```python
from build123d import *

# Parameters (mm, degrees)
SKETCH1_W           = 58.42
SKETCH1_H           = 58.42
BOSS_EXTRUDE1_DEPTH = 56
SKETCH2_R           = 30
BOSS_EXTRUDE2_DEPTH = 72
SKETCH3_R           = 6
BOSS_EXTRUDE3_DEPTH = 30
SKETCH4_R           = 2.5
CUT_EXTRUDE1_DEPTH  = 25.4
SKETCH5_W           = 2.5
SKETCH5_H           = 4
CUT_EXTRUDE2_DEPTH  = 18.8
SKETCH6_R           = 16
BOSS_EXTRUDE4_DEPTH = 2
CUT_EXTRUDE3_REACH  = 28.5


with BuildPart() as part:
    # Sketch1 → Boss-Extrude1 (new body)
    with BuildSketch(Plane(origin=(0, 0, 0), x_dir=(1, 0, 0), z_dir=(0, 1, 0))):
        Rectangle(SKETCH1_W, SKETCH1_H)
    extrude(amount=BOSS_EXTRUDE1_DEPTH)

    # Sketch2 → Boss-Extrude2 (add)
    with BuildSketch(Plane(origin=(0, 56, 0), x_dir=(1, 0, 0), z_dir=(0, 1, 0))):
        Circle(SKETCH2_R)
    extrude(amount=BOSS_EXTRUDE2_DEPTH)

    # Sketch3 → Boss-Extrude3 (add)
    with BuildSketch(Plane(origin=(0, 128, 0), x_dir=(1, 0, 0), z_dir=(0, 1, 0))):
        Circle(SKETCH3_R)
    extrude(amount=BOSS_EXTRUDE3_DEPTH)

    # Sketch4 → Cut-Extrude1 (cut)
    with BuildSketch(Plane(origin=(0, 128, 0), x_dir=(1, 0, 0), z_dir=(0, 1, 0))):
        with Locations((-15.909902577, 15.909902577)):
            Circle(SKETCH4_R)
        with Locations((15.909902577, 15.909902577)):
            Circle(SKETCH4_R)
        with Locations((15.909902577, -15.909902577)):
            Circle(SKETCH4_R)
        with Locations((-15.909902577, -15.909902577)):
            Circle(SKETCH4_R)
    extrude(amount=-CUT_EXTRUDE1_DEPTH, mode=Mode.SUBTRACT)

    # Sketch5 → Cut-Extrude2 (cut)
    with BuildSketch(Plane(origin=(0, 158, 0), x_dir=(1, 0, 0), z_dir=(0, 1, 0))):
        with Locations((4.75, 0)):
            Rectangle(SKETCH5_W, SKETCH5_H)
    extrude(amount=-CUT_EXTRUDE2_DEPTH, mode=Mode.SUBTRACT)

    # Sketch6 → Boss-Extrude4 (add)
    with BuildSketch(Plane(origin=(0, 128, 0), x_dir=(1, 0, 0), z_dir=(0, 1, 0))):
        Circle(SKETCH6_R)
    extrude(amount=BOSS_EXTRUDE4_DEPTH)

    # Sketch7 → Cut-Extrude3 (cut, up to next)
    with BuildSketch(Plane(origin=(3.5, 0, 0), x_dir=(0, 0, -1), z_dir=(1, 0, 0)), mode=Mode.PRIVATE) as cut_extrude3_sk1:
        with BuildLine():
            Line((2, 139.2), (-2, 139.2))
            ThreePointArc((-2, 139.2), (0, 137.2), (2, 139.2))
        make_face()
    cut_extrude3_tool1 = extrude(cut_extrude3_sk1.sketch, amount=CUT_EXTRUDE3_REACH, mode=Mode.PRIVATE) & part.part
    add(cut_extrude3_tool1.solids().sort_by_distance((3.5, 138.351174, 0))[0], mode=Mode.SUBTRACT)


solid = part.part
```
Input: part model. Units: mm. Frame: model coordinates. A direction names the side the tool comes from. Coordinates: 2 decimals unless noted, no trailing zeros. Loops run counter-clockwise (first coordinate to the right, second up) from the corner with the lowest first, then second, coordinate; pieces in that order, holes last. Notation, with made-up numbers: M 62,19 L 112,19 A24 ccw 112,34 Z; hole C 10,65 d4. An arc over 180 degrees is marked long. One line per item, written item: value.
(1) Pin query (flat end, axial travel): pin 1 (4 mm diameter, centred on x = -15.5, y = 93, fed in from +Z); pin 2 (10 mm diameter, centred on x = 7.5, y = 87.5, fed in from -Z); pin 3 (1.2 mm diameter, centred on y = 147.5, z = 1, fed in from +X). Return the tip coordinate at first contact, or that it passes through.
Filled in:
pin 1: z = 26.79
pin 2: z = -29.9
pin 3: x = 3.5
(2) Section A-A (z = 0). Output: boundary loops of the cut face in (x, y), and give its area (3 significant figures).
Filled in:
outline: M -30,56 L -29.21,56 L -29.21,0 L 29.21,0 L 29.21,56 L 30,56 L 30,128 L 16,128 L 16,130 L 6,130 L 6,137.2 L 3.5,137.2 L 3.5,158 L -6,158 L -6,130 L -16,130 L -16,128 L -30,128 Z
area: 7,940 mm^2
(3) Section C-C (y = 23). Output: boundary loops of the cut face in (x, z).
Filled in:
outline: M -29.21,-29.21 L 29.21,-29.21 L 29.21,29.21 L -29.21,29.21 Z
(4) Line query: line 1 along Z through (x, y) = (10, 37.5); line 2 along Z through (x, y) = (14.5, 111); line 3 along Y through (x, z) = (23, -24). Output: solid intervals per line, ascending. Write a range as from..to.
Filled in:
line 1: -29.21..29.21
line 2: -26.26..-17.97, -13.85..13.85, 17.97..26.26
line 3: 0..56
(5) Pull-direction query (X, two-part tool) for faces 1 (the flat face through (3.5, 148, 0)), 2 (the flat face through (13, 128, 13)), 3 (the cylindrical face through (-4.76, 143.8, 3.65)), 4 (the flat face through (-16, 102.6, -16)); classes: +X half, -X half, draft (parallel to the pull), parting line (faces both ways), or undercut.
Filled in:
face 1: +X half
face 2: draft
face 3: parting line
face 4: undercut
(6) Reachability of faces 5 (the cylindrical face through (-3.47, 128.99, 15.62)), 6 (the flat face through (0, 28, 29.21)), 7 (the flat face through (-23, 56, 24)) from +Z, -Z, +X, -X, +Y, -Y: full face, straight path, thin tool, end or side. Return the list, or none.
Filled in:
face 5: +Y
face 6: +Z, +X, -X, -Y
face 7: +Z, -X, +Y
(7) Section D-D (z = -26). Output: boundary loops of the cut face in (x, y).
Filled in:
outline: M -29.21,0 L 29.21,0 L 29.21,56 L 14.97,56 L 14.97,128 L -14.97,128 L -14.97,56 L -29.21,56 Z
(8) Section B-B (x = 0). Output: boundary loops of the cut face in (y, z), and give its area (3 significant figures).
Filled in:
outline: M 0,-29.21 L 56,-29.21 L 56,-30 L 128,-30 L 128,-16 L 130,-16 L 130,-6 L 158,-6 L 158,6 L 130,6 L 130,16 L 128,16 L 128,30 L 56,30 L 56,29.21 L 0,29.21 Z
area: 7,990 mm^2
